from build123d import *

# Parameters (mm, degrees)
BARS_START           = -20.4
BARS_DEPTH           = 40.8
BARS_2_DEPTH         = 40.8
BARS_3_DEPTH         = 40.8
BARS_4_DEPTH         = 40.8
BARS_5_DEPTH         = 40.8
BARS_6_DEPTH         = 40.8
BARS_7_DEPTH         = 40.8
BARS_8_DEPTH         = 40.8
BARS_9_DEPTH         = 40.8
BARS_10_DEPTH        = 40.8
BARS_11_DEPTH        = 40.8
BARS_12_DEPTH        = 40.8
BARS_13_DEPTH        = 40.8
BARS_14_DEPTH        = 40.8
BARS_15_DEPTH        = 40.8
BARS_16_DEPTH        = 40.8
BARS_17_DEPTH        = 40.8
BARS_18_DEPTH        = 40.8
BARS_19_DEPTH        = 40.8
BARS_20_DEPTH        = 40.8
BARS_21_DEPTH        = 40.8
BARS_22_DEPTH        = 40.8
BARS_23_DEPTH        = 40.8
BARS_24_DEPTH        = 40.8
BARS_25_DEPTH        = 40.8
BARS_26_DEPTH        = 40.8
BARS_27_DEPTH        = 40.8
BARS_28_DEPTH        = 40.8
BARS_29_DEPTH        = 40.8
END_RING_FRONT_START = 20.3
SKETCH_2_R           = 30
SKETCH_2_R_2         = 22.4
END_RING_FRONT_DEPTH = 6
END_RING_REAR_START  = -26.3
SKETCH_3_R           = 30
SKETCH_3_R_2         = 22.4
END_RING_REAR_DEPTH  = 6


with BuildPart() as part:
    # Эскиз1 → Bars (new body)
    with BuildSketch(Plane.XY.offset(BARS_START)):
        Polygon((22.533161901, 0.262896843), (28.918731651, 0.692430264), (28.750945159, 3.186793448), (22.365375408, 2.757260027), align=None)
    extrude(amount=BARS_DEPTH)



with BuildPart() as body_2:
    # Эскиз1 → Bars 2 (new body)
    with BuildSketch(Plane.XY.offset(BARS_START)):
        Polygon((21.949834048, 5.100714194), (28.093775737, 6.892914103), (27.393697648, 9.292891325), (21.249755958, 7.500691416), align=None)
    extrude(amount=BARS_2_DEPTH)


with BuildPart() as body_3:
    # Эскиз1 → Bars 3 (new body)
    with BuildSketch(Plane.XY.offset(BARS_START)):
        Polygon((20.34015635, 9.700027818), (25.955186093, 12.771092939), (24.755551281, 14.964463933), (19.140521537, 11.893398812), align=None)
    extrude(amount=BARS_3_DEPTH)


with BuildPart() as body_4:
    # Эскиз1 → Bars 4 (new body)
    with BuildSketch(Plane.XY.offset(BARS_START)):
        Polygon((17.779395547, 13.845778923), (22.602960795, 18.052109663), (20.959862849, 19.936314838), (16.136297602, 15.729984098), align=None)
    extrude(amount=BARS_4_DEPTH)


with BuildPart() as body_5:
    # Эскиз1 → Bars 5 (new body)
    with BuildSketch(Plane.XY.offset(BARS_START)):
        Polygon((14.387289969, 17.344116793), (18.193846171, 22.489029803), (16.184114527, 23.97596582), (12.377558325, 18.83105281), align=None)
    extrude(amount=BARS_5_DEPTH)


with BuildPart() as body_6:
    # Эскиз1 → Bars 6 (new body)
    with BuildSketch(Plane.XY.offset(BARS_START)):
        Polygon((10.322450703, 20.031463039), (12.934007522, 25.874387904), (10.651614996, 26.894527287), (8.040058177, 21.051602421), align=None)
    extrude(amount=BARS_6_DEPTH)


with BuildPart() as body_7:
    # Эскиз1 → Bars 7 (new body)
    with BuildSketch(Plane.XY.offset(BARS_START)):
        Polygon((5.774945114, 21.782160337), (7.069389055, 28.049888385), (4.621057787, 28.555530549), (3.326613846, 22.287802501), align=None)
    extrude(amount=BARS_7_DEPTH)


with BuildPart() as body_8:
    # Эскиз1 → Bars 8 (new body)
    with BuildSketch(Plane.XY.offset(BARS_START)):
        Polygon((0.95740951, 22.514348026), (0.874213814, 28.913807259), (-1.625574949, 28.88130894), (-1.542379252, 22.481849707), align=None)
    extrude(amount=BARS_8_DEPTH)


with BuildPart() as body_9:
    # Эскиз1 → Bars 9 (new body)
    with BuildSketch(Plane.XY.offset(BARS_START)):
        Polygon((-3.904893498, 22.193789824), (-5.361838694, 28.425748641), (-7.796197607, 27.856629424), (-6.339252411, 21.624670607), align=None)
    extrude(amount=BARS_9_DEPTH)


with BuildPart() as body_10:
    # Эскиз1 → Bars 10 (new body)
    with BuildSketch(Plane.XY.offset(BARS_START)):
        Polygon((-8.584608027, 20.835474677), (-11.347177584, 26.60853361), (-13.602278729, 25.529404877), (-10.839709172, 19.756345944), align=None)
    extrude(amount=BARS_10_DEPTH)


with BuildPart() as body_11:
    # Эскиз1 → Bars 11 (new body)
    with BuildSketch(Plane.XY.offset(BARS_START)):
        Polygon((-12.862915825, 18.502915891), (-16.801935061, 23.547133121), (-18.772332416, 22.008453732), (-14.83331318, 16.964236502), align=None)
    extrude(amount=BARS_11_DEPTH)


with BuildPart() as body_12:
    # Эскиз1 → Bars 12 (new body)
    with BuildSketch(Plane.XY.offset(BARS_START)):
        Polygon((-16.539767975, 15.305181323), (-21.471052729, 19.384694857), (-23.064612703, 17.45841175), (-18.13332795, 13.378898216), align=None)
    extrude(amount=BARS_12_DEPTH)


with BuildPart() as body_13:
    # Эскиз1 → Bars 13 (new body)
    with BuildSketch(Plane.XY.offset(BARS_START)):
        Polygon((-19.443238958, 11.391793486), (-25.136207835, 14.315849807), (-26.278417335, 12.092033839), (-20.585448458, 9.167977519), align=None)
    extrude(amount=BARS_13_DEPTH)


with BuildPart() as body_14:
    # Эскиз1 → Bars 14 (new body)
    with BuildSketch(Plane.XY.offset(BARS_START)):
        Polygon((-21.437565696, 6.945738047), (-27.626021799, 8.57761153), (-28.263472378, 6.160245865), (-22.075016276, 4.528372382), align=None)
    extrude(amount=BARS_14_DEPTH)


with BuildPart() as body_15:
    # Эскиз1 → Bars 15 (new body)
    with BuildSketch(Plane.XY.offset(BARS_START)):
        Polygon((-22.429495689, 2.174907617), (-28.824073688, 2.438293672), (-28.926958866, -0.059588359), (-22.532380867, -0.322974414), align=None)
    extrude(amount=BARS_15_DEPTH)


with BuildPart() as body_16:
    # Эскиз1 → Bars 16 (new body)
    with BuildSketch(Plane.XY.offset(BARS_START)):
        Polygon((-22.372647392, -2.697619077), (-28.674343927, -3.815036088), (-28.237852907, -6.276636298), (-21.936156372, -5.159219286), align=None)
    extrude(amount=BARS_16_DEPTH)


with BuildPart() as body_17:
    # Эскиз1 → Bars 17 (new body)
    with BuildSketch(Plane.XY.offset(BARS_START)):
        Polygon((-21.269678968, -7.4440081), (-27.183833713, -9.889979002), (-26.22837633, -12.200195699), (-20.314221585, -9.754224798), align=None)
    extrude(amount=BARS_17_DEPTH)


with BuildPart() as body_18:
    # Эскиз1 → Bars 18 (new body)
    with BuildSketch(Plane.XY.offset(BARS_START)):
        Polygon((-19.172163995, -11.842323579), (-24.422237648, -15.502477488), (-22.992490027, -17.553287509), (-17.742416374, -13.893133599), align=None)
    extrude(amount=BARS_18_DEPTH)


with BuildPart() as body_19:
    # Эскиз1 → Bars 19 (new body)
    with BuildSketch(Plane.XY.offset(BARS_START)):
        Polygon((-16.178179942, -15.686905168), (-20.518684893, -20.390097358), (-18.681500444, -22.085607104), (-14.340995493, -17.382414915), align=None)
    extrude(amount=BARS_19_DEPTH)


with BuildPart() as body_20:
    # Эскиз1 → Bars 20 (new body)
    with BuildSketch(Plane.XY.offset(BARS_START)):
        Polygon((-12.427722176, -18.797984507), (-15.655701238, -24.324298936), (-13.496984664, -25.585228257), (-10.269005602, -20.058913828), align=None)
    extrude(amount=BARS_20_DEPTH)


with BuildPart() as body_21:
    # Эскиз1 → Bars 21 (new body)
    with BuildSketch(Plane.XY.offset(BARS_START)):
        Polygon((-8.096157933, -21.030090982), (-10.060674393, -27.121123332), (-7.681364881, -27.888512573), (-5.716848422, -21.797480224), align=None)
    extrude(amount=BARS_21_DEPTH)


with BuildPart() as body_22:
    # Эскиз1 → Bars 22 (new body)
    with BuildSketch(Plane.XY.offset(BARS_START)):
        Polygon((-3.386026344, -22.278853777), (-3.995221595, -28.649794143), (-1.506573014, -28.887761037), (-0.897377763, -22.516820671), align=None)
    extrude(amount=BARS_22_DEPTH)


with BuildPart() as body_23:
    # Эскиз1 → Bars 23 (new body)
    with BuildSketch(Plane.XY.offset(BARS_START)):
        Polygon((1.482432074, -22.48588213), (2.257043325, -28.838832421), (4.738664533, -28.536249902), (3.964053282, -22.18329961), align=None)
    extrude(amount=BARS_23_DEPTH)


with BuildPart() as body_24:
    # Эскиз1 → Bars 24 (new body)
    with BuildSketch(Plane.XY.offset(BARS_START)):
        Polygon((6.281573616, -21.641495625), (8.403771407, -27.679398948), (10.762327392, -26.850415436), (8.640129601, -20.812512113), align=None)
    extrude(amount=BARS_24_DEPTH)


with BuildPart() as body_25:
    # Эскиз1 → Bars 25 (new body)
    with BuildSketch(Plane.XY.offset(BARS_START)):
        Polygon((10.786995757, -19.785176839), (14.157548478, -25.225707544), (16.282755785, -23.909085387), (12.912203064, -18.468554682), align=None)
    extrude(amount=BARS_25_DEPTH)


with BuildPart() as body_26:
    # Эскиз1 → Bars 26 (new body)
    with BuildSketch(Plane.XY.offset(BARS_START)):
        Polygon((14.788029965, -17.003725173), (19.249334318, -21.592490091), (21.041820614, -19.849793078), (16.580516262, -15.26102816), align=None)
    extrude(amount=BARS_26_DEPTH)


with BuildPart() as body_27:
    # Эскиз1 → Bars 27 (new body)
    with BuildSketch(Plane.XY.offset(BARS_START)):
        Polygon((18.097592328, -13.427198216), (23.441042678, -16.9496318), (24.816993297, -14.862346507), (19.473542947, -11.339912923), align=None)
    extrude(amount=BARS_27_DEPTH)


with BuildPart() as body_28:
    # Эскиз1 → Bars 28 (new body)
    with BuildSketch(Plane.XY.offset(BARS_START)):
        Polygon((20.560931388, -9.222830393), (26.536673936, -11.514227564), (27.431750956, -9.179953131), (21.456008407, -6.88855596), align=None)
    extrude(amount=BARS_28_DEPTH)


with BuildPart() as body_29:
    # Эскиз1 → Bars 29 (new body)
    with BuildSketch(Plane.XY.offset(BARS_START)):
        Polygon((22.062864148, -4.587213273), (28.391479815, -5.540430844), (28.763830428, -3.068315349), (22.435214761, -2.115097778), align=None)
    extrude(amount=BARS_29_DEPTH)


with BuildPart() as part_1:
    add(part.part)

    add(body_2.part)  # End_ring_front merges body 2

    add(body_3.part)  # End_ring_front merges body 3

    add(body_4.part)  # End_ring_front merges body 4

    add(body_5.part)  # End_ring_front merges body 5

    add(body_6.part)  # End_ring_front merges body 6

    add(body_7.part)  # End_ring_front merges body 7

    add(body_8.part)  # End_ring_front merges body 8

    add(body_9.part)  # End_ring_front merges body 9

    add(body_10.part)  # End_ring_front merges body 10

    add(body_11.part)  # End_ring_front merges body 11

    add(body_12.part)  # End_ring_front merges body 12

    add(body_13.part)  # End_ring_front merges body 13

    add(body_14.part)  # End_ring_front merges body 14

    add(body_15.part)  # End_ring_front merges body 15

    add(body_16.part)  # End_ring_front merges body 16

    add(body_17.part)  # End_ring_front merges body 17

    add(body_18.part)  # End_ring_front merges body 18

    add(body_19.part)  # End_ring_front merges body 19

    add(body_20.part)  # End_ring_front merges body 20

    add(body_21.part)  # End_ring_front merges body 21

    add(body_22.part)  # End_ring_front merges body 22

    add(body_23.part)  # End_ring_front merges body 23

    add(body_24.part)  # End_ring_front merges body 24

    add(body_25.part)  # End_ring_front merges body 25

    add(body_26.part)  # End_ring_front merges body 26

    add(body_27.part)  # End_ring_front merges body 27

    add(body_28.part)  # End_ring_front merges body 28

    add(body_29.part)  # End_ring_front merges body 29
    # Эскиз2 → End_ring_front (add)
    with BuildSketch(Plane.XY.offset(END_RING_FRONT_START)):
        Circle(SKETCH_2_R)
        Circle(SKETCH_2_R_2, mode=Mode.SUBTRACT)
    extrude(amount=END_RING_FRONT_DEPTH)

    # Эскиз3 → End_ring_rear (add)
    with BuildSketch(Plane.XY.offset(END_RING_REAR_START)):
        Circle(SKETCH_3_R)
        Circle(SKETCH_3_R_2, mode=Mode.SUBTRACT)
    extrude(amount=END_RING_REAR_DEPTH)


solid = part_1.part
Can you work these out from the model? Positions are in its coordinate system, mm. A direction names the side the tool comes from. Give positions to 0.01 mm unless a question says otherwise; leave off trailing zeros. Loops run counter-clockwise (first coordinate to the right, second up) from the corner with the lowest first, then second, coordinate; pieces in that order, holes last. Notation, with made-up numbers: (32, 84.25) - (67, 84.25) arc R20 ccw to (67, 94.25) - close; hole circle Ø2 at (24.5, -36). An arc over 180 degrees is marked (long way). One line per item, written item: value.
(1) If we section it at B-B, the plane z = 6: State how many separate pieces and enclosed holes the cut face has, plus the area to 3 significant figures.
Verdict:
separate pieces: 29
enclosed holes: 0
area: 464 mm^2
(2) I'm going to push flat-ended pins straight in: pin 1 (8 mm diameter, centred on x = -20.5, z = 3.5, fed in from -Y); pin 2 (5 mm diameter, centred on y = -3.5, z = 20.5, fed in from -X); pin 3 (8 mm diameter, centred on y = 5.5, z = 7.5, fed in from -X). Where does each tip first touch, or does it pass through?
Verdict:
pin 1: y = -22.09
pin 2: x = -29.98
pin 3: x = -28.86
(3) On a 3-axis mill with a long thin cutter (end or side, diameter ignored), from which of +Z, -Z, +X, -X, +Y, -Y can I reach the whole of each face in a straight line? I mean faces 1 (the face through (3.983, 25.466, -0.284)), 2 (the face through (-6.713, -24.886, -0.284)), 3 (the face through (-22.15, -3.95, -0.28)). Say none if no direction works.
Verdict:
face 1: +Y
face 2: -Y
face 3: none
(4) If we section it at A-A, the plane x = 0: List the corners of the cut face in (y, z) for me, plus the area to 3 significant figures.
Verdict:
outline: (-30, -26.3) - (-22.4, -26.3) - (-22.4, -20.3) - (-30, -20.3) - close; (-30, 20.3) - (-22.4, 20.3) - (-22.4, 26.3) - (-30, 26.3) - close; (22.4, -26.3) - (30, -26.3) - (30, -20.3) - (28.9, -20.3) - (28.9, 20.3) - (30, 20.3) - (30, 26.3) - (22.4, 26.3) - (22.4, 20.3) - (22.5, 20.3) - (22.5, -20.3) - (22.4, -20.3) - close
area: 442 mm^2
(5) I need wall thicknesses on line 1 along Y through (x, z) = (0, -24.2); line 2 along X through (y, z) = (14, -4); line 3 along X through (y, z) = (-25, -2.5). Which ranges of each line are inside material? Lowest first, please.
Verdict:
line 1: -30 to -22.4, 22.4 to 30
line 2: -25.3 to -24.52, -18.88 to -17.62, 17.64 to 17.96, 22.99 to 25.28
line 3: -14.5 to -13.16, -9.38 to -6.75, -3.65 to -1.13, 1.79 to 4.31, 7.46 to 10.11, 14.02 to 14.52
